Can you work these out from the drawing? Everything is in mm from the part's minimum corner. Give positions to 0.01 mm unless a question says otherwise; leave off trailing zeros. Loops run counter-clockwise (first coordinate to the right, second up) from the corner with the lowest first, then second, coordinate; pieces in that order, holes last. Notation, with made-up numbers: (13, -21.75) -> (18, -21.75) arc R24 cw to (18, -5.75) -> close; hole circle Ø6 at (-3.5, 4.25). An arc over 180 degrees is marked (long way). Return JSON: item names as keys, results as strings. Group by question number.
Q1. Suppose I cut it at C-C, the plane z = 15.25. Please give me the cut outline in (x, y), and give its area (3 significant figures).
Q2. I need wall thicknesses on line 1 along Y through (x, z) = (20, 10); line 2 along Y through (x, z) = (20, 2.9); line 3 along Z through (x, y) = (15, 28). Which ranges of each line are inside material? Lowest first, please. Write a range as [from, to].
Q3. Will these pins go through, and if not, where does the flat tip stop? pin 1 (4 mm diameter, centred on y = 33.5, z = 7.5, fed in from -X); pin 2 (6.5 mm diameter, centred on x = 20, y = 20, fed in from -Z); pin 3 (12 mm diameter, centred on x = 33, y = 18.5, fed in from +Z); pin 4 (4 mm diameter, centred on x = 12, z = 16, fed in from -Y).
Q4. Suppose I cut it at A-A, the plane x = 20. Please give me the cut outline in (y, z).
Q5. Thinking about a two-plate mould opening in Y: for the marked faces 1, 2 and 3, which applies, pulls with the +Y half, pulls with the -Y half, needs draft (parallel to the pull), parting line crosses it, or undercut?
Q6. Suppose I cut it at D-D, the plane y = 15.5. Please give me the cut outline in (x, z), and give its area (3 significant figures).
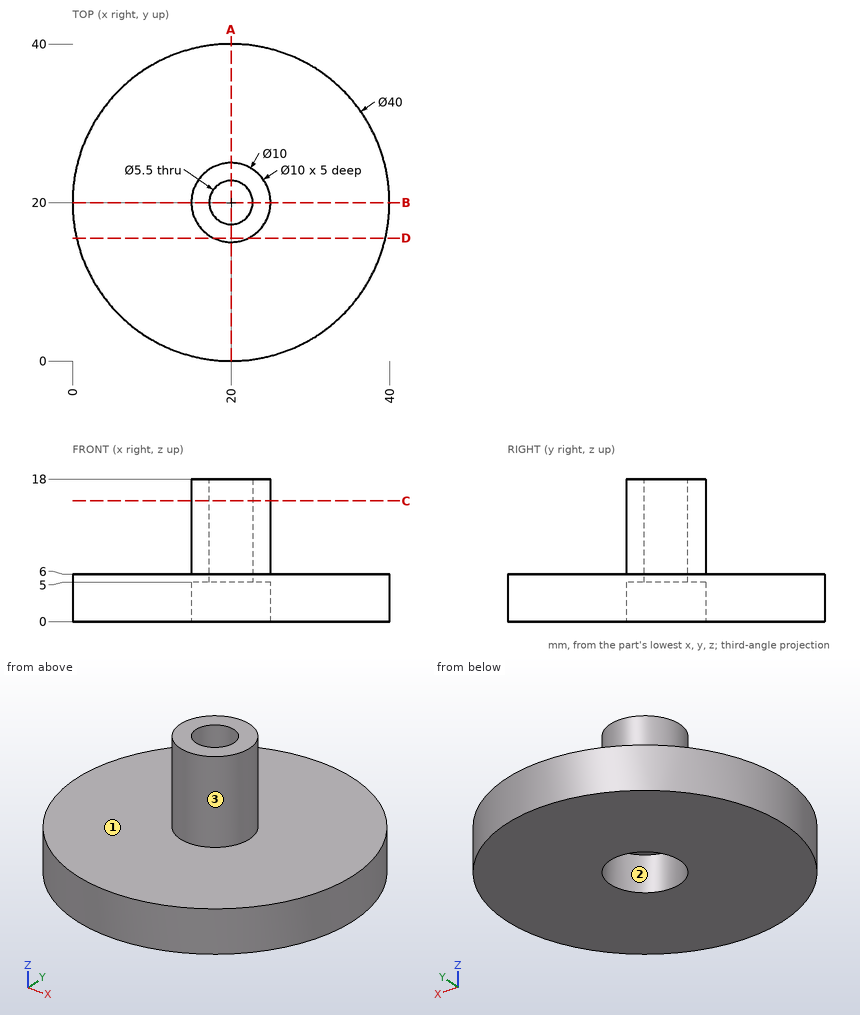
Ans:
{
 "1": {"outline": "circle Ø10 at (20, 20); hole circle Ø5.5 at (20, 20)", "area": "54.8 mm^2"},
 "2": {"line 1": "y = [15, 17.25], [22.75, 25]", "line 2": "y = [0, 15], [25, 40]", "line 3": "z = [0, 6]"},
 "3": {"pin 1": "stops at x = 4.13", "pin 2": "stops at z = 5", "pin 3": "stops at z = 6", "pin 4": "passes through"},
 "4": {"outline": "(0, 0) -> (15, 0) -> (15, 5) -> (17.25, 5) -> (17.25, 18) -> (15, 18) -> (15, 6) -> (0, 6) -> close; (22.75, 5) -> (25, 5) -> (25, 0) -> (40, 0) -> (40, 6) -> (25, 6) -> (25, 18) -> (22.75, 18) -> close"},
 "5": {"face 1": "needs draft", "face 2": "undercut", "face 3": "parting line crosses it"},
 "6": {"outline": "(0.51, 0) -> (17.82, 0) -> (17.82, 5) -> (22.18, 5) -> (22.18, 0) -> (39.49, 0) -> (39.49, 6) -> (22.18, 6) -> (22.18, 18) -> (17.82, 18) -> (17.82, 6) -> (0.51, 6) -> close", "area": "264 mm^2"}
}
